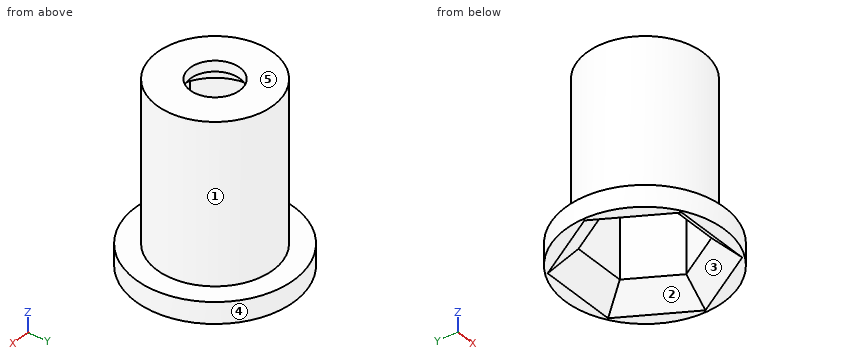
Autodesk Inventor part; units mm, degrees
ref_plane "YZ Plane" through (0, 0, 0) normal (1, 0, 0) x (0, 1, 0)
ref_plane "XZ Plane" through (0, 0, 0) normal (0, 1, 0) x (-1, 0, 0)
ref_plane "XY Plane" through (0, 0, 0) normal (0, 0, 1) x (1, 0, 0)
sketch "Sketch2" plane through (0, 0, 0) normal (0, 0, 1) x (1, 0, 0)
  circle A0 centre (0, 0) radius 7.5
  dimension "d0" = 15
extrude "Extrusion1" add sketch "Sketch2" along normal blind 2
sketch "Sketch3" plane through (0, 0, 2) normal (0, 0, 1) x (1, 0, 0)
  circle A0 centre (0, 0) radius 7.5
  circle A1 centre (0, 0) radius 5.5
  dimension "d3" = 11
extrude "Extrusion2" add sketch "Sketch3" along normal blind 15 contours A1
sketch "Sketch4" plane through (0, 0, 0) normal (0, 0, -1) x (-1, 0, 0)
  circle A0 centre (0, 0) radius 7.5
hole "Hole1" at (0, 0, 0) direction (0, 0, 1) diameter 4.7 end through all
ref_plane "Work Plane1" through (0, 0, 16) normal (0, 0, 1) x (1, 0, 0)
sketch "Sketch5" plane through (0, 0, 0) normal (0, 0, -1) x (-1, 0, 0)
  circle A0 centre (0, 0) radius 2.35
  circle A1 centre (0, 0) radius 7.5
  line L0 (2.4934, 4.3187) -> (4.9869, 0)
  line L1 (4.9869, 0) -> (2.4934, -4.3188)
  line L2 (2.4934, -4.3188) -> (-2.4934, -4.3187)
  line L3 (-2.4934, -4.3187) -> (-4.9869, 0)
  line L4 (-4.9869, 0) -> (-2.4934, 4.3187)
  line L5 (-2.4934, 4.3187) -> (2.4934, 4.3187)
  dimension "d14" = 8.6375
extrude "Extrusion3" cut sketch "Sketch5" against normal up to surface (16 mm away) contours L0 L1 L2 L3 L4 L5
sketch "Sketch6" plane through (0, 0, 0) normal (0, 0, -1) x (-1, 0, 0)
  line L0 (2.4934, -4.3188) -> (-2.4934, -4.3187)
  line L1 (-2.4934, -4.3187) -> (-4.9869, 0)
  line L2 (-4.9869, 0) -> (-2.4934, 4.3187)
  line L3 (-2.4934, 4.3187) -> (2.4934, 4.3187)
  line L4 (2.4934, 4.3187) -> (4.9869, 0)
  line L5 (4.9869, 0) -> (2.4934, -4.3188)
  circle A0 centre (0, 0) radius 7.5
  circle A1 centre (0, 0) radius 4 construction
  dimension "d17" = 8
sketch "Sketch7" plane through (0, 0, 0) normal (1, 0, 0) x (0, 1, 0)
  line L0 (-7.5, 0) -> (-7.5, 2)
  line L1 (-7.5, 2) -> (-5.5, 2)
  line L2 (-5.5, 2) -> (-5.5, 17)
  line L3 (-5.5, 17) -> (-2.35, 17)
  line L4 (-2.35, 17) -> (-2.35, 16)
  line L5 (-2.35, 16) -> (-4.3187, 16)
  line L6 (-4.3187, 16) -> (-4.3187, 0)
  line L7 (-4.3187, 0) -> (-7.5, 0)
  line L8 (7.5, 2) -> (7.5, 0)
  line L9 (7.5, 0) -> (4.3187, 0)
  line L10 (4.3187, 0) -> (4.3187, 16)
  line L11 (4.3187, 16) -> (2.35, 16)
  line L12 (2.35, 16) -> (2.35, 17)
  line L13 (2.35, 17) -> (5.5, 17)
  line L14 (5.5, 17) -> (5.5, 2)
  line L15 (5.5, 2) -> (7.5, 2)
  line L16 (2.35, 16) -> (4.3187, 14.0313)
  line L17 (0, -3.4) -> (0, 20.4)
  point P0 (0, 0)
  dimension "d18" = 45
revolve "Revolution1" add sketch "Sketch7" angle 360 about axis through (0, 0, -10) along (0, 0, 1) contours L16 L11 L10
chamfer "Chamfer1" distance 2 angle 45 6 edges at (0, -4.3187, 0) (3.7401, -2.1594, 0) (3.7401, 2.1594, 0) (0, 4.3187, 0) (-3.7401, 2.1594, 0) (-3.7401, -2.1594, 0)
properties part number "z-keeper"
Design review of the part built by this model. Coordinates are the model's own, in mm. Face numbers are marked on the shaded views. A direction names the side the tool comes from. Give positions to 0.01 mm unless a question says otherwise; leave off trailing zeros. Order: outer loops, then holes, each group sorted by start corner. A loop starts at its lowest first (then second) coordinate and runs counter-clockwise, first axis right, second up. Notation, with made-up numbers: (24.25, -18) - (55.25, -18) arc R30 cw to (55.25, 5) - close; hole circle Ø11 at (30, -20). An arc over 180 degrees is marked (long way). Write item = value, one per line. Start each with the question number.
Q1. Tool access review of the marked faces 1 and 2: name each direction out of +Z, -Z, +X, -X, +Y, -Y from which nothing blocks a thin tool from reaching the whole face with its end or side.
Q2. We need section A-A on z = 14.5. State the section outline as (x, y) points.
Q3. To check wall thickness, follow L1, parallel to Y at x = 0, z = 16.35; L2, parallel to Y at x = 0, z = 10; L3, parallel to X at y = 3.5, z = 13. State the ranges of each line that lie inside material, in increasing order. Write a range as from..to.
Q4. We need section B-B on z = 6. State the section outline as (x, y) points, plus the area to 3 significant figures.
Q5. Mouldability with a two-part tool opening along Y and no side actions: class the marked faces 3, 4 and 5 as released by +Y, released by -Y, zero draft, split by the parting line, or undercut.
Q6. We need section C-C on y = 4.75. State the section outline as (x, z) points, plus the area to 4 significant figures.
Q7. Clearance check with flat-ended pins moving along their axes: pin 1 Ø5 at (x, z) = (6, 3) entering from +Y; pin 2 Ø5 at (y, z) = (-0.5, 11) entering from +X; pin 3 Ø1 at (x, y) = (-0.5, 1.5) entering from +Z; pin 4 Ø4 at (x, z) = (0.5, 10) entering from +Y. State where each tip first meets the part, or that it passes through.
Working result:
q1.face_1 = +Z
q1.face_2 = -Z
q2.outline = circle Ø11 at (0, 0); circle Ø8.64 at (0, 0); hole (-4.99, 0) - (-2.49, -4.32) - (2.49, -4.32) - (4.99, 0) - (2.49, 4.32) - (-2.49, 4.32) - close; hole circle Ø7.7 at (0, 0)
q3.L1 = -5.5..-2.35, 2.35..5.5
q3.L2 = -5.5..-4.32, 4.32..5.5
q3.L3 = -4.24..-2.97, 2.97..4.24
q4.outline = circle Ø11 at (0, 0); hole (-4.99, 0) - (-2.49, -4.32) - (2.49, -4.32) - (4.99, 0) - (2.49, 4.32) - (-2.49, 4.32) - close
q4.area = 30.4 mm²
q5.face_3 = undercut
q5.face_4 = split by the parting line
q5.face_5 = zero draft
q6.outline = (-5.8, 0) - (-4.55, 0) - (-2.74, 1.57) - (2.74, 1.57) - (4.55, 0) - (5.8, 0) - (5.8, 2) - (2.77, 2) - (2.77, 17) - (-2.77, 17) - (-2.77, 2) - (-5.8, 2) - close
q6.area = 94.95 mm²
q7.pin_1 = 6.52
q7.pin_2 = 5.5
q7.pin_3 = through
q7.pin_4 = 5.5
